Check sheet for the modelled part. Datum: model origin and axes. Units: mm. A direction names the side the tool comes from. Round coordinates to 2 decimals unless told otherwise and drop trailing zeros. Write each loop counter-clockwise with the first axis right and the second up, starting at its lowest first coordinate (ties: lowest second). Pieces come first, ordered by that corner, then holes.
Item 1: Cross-section at A-A on z = 12. Enter the section's corners in (x, y).
Item 2: Release check for a two-part mould opening along Z. For faces 1 (the flat face through (13.7, 2.8, 28.2)), 2 (the flat face through (7, 3, 0)), 3 (the flat face through (5, 0.45, 49)) record: +Z half, -Z half, draft (parallel to the pull), parting line (faces both ways), or undercut.
Item 3: Go/stop test with flat-tipped pins: pin 1 Ø0.5 at (y, z) = (0, 49) entering from +X; pin 2 Ø0.7 at (x, z) = (4.5, 43) entering from -Y; pin 3 Ø7.5 at (x, z) = (8.5, 34) entering from +Y. Record where each tip stops, or that it passes through.
Item 4: Tool access check on faces 4 (the flat face through (13.7, 2.8, 8.2)), 5 (the flat face through (6.995, -2.047, 50.675)), 6 (the flat face through (13, 2, 6.45)). Record the directions out of +Z, -Z, +X, -X, +Y, -Y that give a thin tool (end or side, any length) a straight path to the whole face; none if there is none.
Item 5: Material ranges on line 1 (Z direction, x = 12.25, y = 2.75); line 2 (Y direction, x = 11, z = 83.5); line 3 (Y direction, x = 9, z = 69), recorded low to high.
from build123d import *

# Parameters (mm, degrees)
BOSS_EXTRUDE1_DEPTH = 99.95
BOSS_EXTRUDE2_DEPTH = 99.95
SKETCH3_R           = 2.3
CUT_EXTRUDE1_DEPTH  = 203
SKETCH4_W           = 3.5
SKETCH4_H           = 4
CUT_EXTRUDE2_DEPTH  = 3
LPATTERN1_COUNT     = 10
LPATTERN1_PITCH     = 20
THICKEN1_T1         = 2
THICKEN2_T1         = 2
BOSS_EXTRUDE3_DEPTH = 99.95
CHAMFER1_SIZE       = 4.717915225
CHAMFER1_SIZE_2     = 2.2
CHAMFER2_SIZE       = 2.2


with BuildPart() as part:
    # Sketch1 → Boss-Extrude1 (new body)
    with BuildSketch(Plane.XY):
        with BuildLine():
            Line((0, 0.393921198), (0, 5.406078802))
            ThreePointArc((0, 5.406078802), (0.08229014, 5.759480212), (0.312231391, 6.040177993))
            Line((0.312231391, 6.040177993), (2.612231391, 7.809408763))
            ThreePointArc((2.612231391, 7.809408763), (3.45340141, 7.893019432), (3.9, 7.175309571))
            Line((3.9, 7.175309571), (3.9, 5.35))
            Line((3.9, 5.35), (6.3, 5.35))
            Line((6.3, 5.35), (6.3, 0.45))
            Line((6.3, 0.45), (3.9, 0.45))
            Line((3.9, 0.45), (3.9, -1.375309571))
            ThreePointArc((3.9, -1.375309571), (3.45340141, -2.093019432), (2.612231391, -2.009408763))
            Line((2.612231391, -2.009408763), (0.312231391, -0.240177993))
            ThreePointArc((0.312231391, -0.240177993), (0.08229014, 0.040519788), (0, 0.393921198))
        make_face()
    extrude(amount=BOSS_EXTRUDE1_DEPTH)

    # Sketch2 → Boss-Extrude2 (add)
    with BuildSketch(Plane.XY.offset(99.95)):
        Polygon((17.472453889, 5.35), (6.3, 5.35), (6.3, 0.45), (9.987087866, -4.283432483), (10.933774362, -3.54601491), (9.831668963, -2.122862181), (17.26318939, 3.66589025), (18.369311325, 2.245866185), (19.315997822, 2.983283759), align=None)
    extrude(amount=-BOSS_EXTRUDE2_DEPTH)

    # Sketch3 → Cut-Extrude1 (cut)
    with BuildSketch(Plane.XY.offset(99.95)):
        with Locations((9.9, 1.95)):
            Circle(SKETCH3_R)
    extrude(amount=-CUT_EXTRUDE1_DEPTH, mode=Mode.SUBTRACT)

    # Sketch4 → Cut-Extrude2 (cut)
    with BuildSketch(Plane(origin=(6.0943119, -5.034061174, 0), x_dir=(0, 0, -1), z_dir=(0.6145146443247225, -0.7889054137920846, 0))):
        with Locations((-88.2, 8.814603366)):
            Rectangle(SKETCH4_W, SKETCH4_H)
    cut_extrude2 = extrude(amount=-CUT_EXTRUDE2_DEPTH, mode=Mode.SUBTRACT)

    # LPattern1: Cut-Extrude2 ×10
    with Locations(*[(0, 0, -i * LPATTERN1_PITCH) for i in range(1, LPATTERN1_COUNT)]):
        add(cut_extrude2, mode=Mode.SUBTRACT)

    # Surface-Offset1: a surface, a copy of 1 face of the part
    surface_offset1_1 = part.part.faces().sort_by_distance((10.460431114, -3.914723696, 49.975))[0]
    add(Solid.thicken(surface_offset1_1, THICKEN1_T1))

    # Surface-Offset2: a surface, a copy of 1 face of the part
    surface_offset2_2 = part.part.faces().sort_by_distance((18.842654573, 2.614574972, 49.975))[0]
    add(Solid.thicken(surface_offset2_2, THICKEN2_T1))

    # Sketch5 → Boss-Extrude3 (add)
    with BuildSketch(Plane.XY.offset(99.95)):
        Polygon((11.216117155, -5.86124331), (9.638306327, -7.090272599), (7.794762394, -4.723556358), (9.372573222, -3.494527069), align=None)
        Polygon((22.126854473, 2.637630884), (20.28331054, 5.004347125), (17.754796681, 3.034771599), (19.598340614, 0.668055358), align=None)
    extrude(amount=-BOSS_EXTRUDE3_DEPTH)

    # Chamfer1
    # the kernel refuses this chamfer: 4.717915225, 2.2 mm, written as the material it adds along each edge
    with BuildSketch(Plane(origin=(9.372573222, -3.494527069, 99.95), x_dir=(-0.6015649261356993, 0.7988239102852083, 0), z_dir=(0, 0, -1))) as chamfer1_piece_1_section:
        Polygon((CHAMFER1_SIZE * 0.999866964139, -CHAMFER1_SIZE * 0.0163111641315), (-CHAMFER1_SIZE_2 * 0.0163111641311, -CHAMFER1_SIZE_2 * 0.999866964113), (0, 0), align=None)
    chamfer1_piece_1 = extrude(amount=99.95, mode=Mode.PRIVATE)
    chamfer1_piece_1 = split(chamfer1_piece_1, bisect_by=Plane(origin=(6.797025318, -3.442675278, 49.975), z_dir=(0.7889054137920843, 0.6145146443247225, 0)), keep=Keep.TOP, mode=Mode.PRIVATE)
    add(chamfer1_piece_1)

    # Chamfer2
    # the kernel refuses this chamfer: 2.2 mm, written as the material it adds along each edge
    with BuildSketch(Plane(origin=(18.701483177, 3.772189172, 0), x_dir=(-0.6359739526449933, 0.7717105231607922, 0), z_dir=(0, 0, 1))) as chamfer2_piece_1_section:
        Polygon((CHAMFER2_SIZE * 0.999621916911, -CHAMFER2_SIZE * 0.0274958766106), (-CHAMFER2_SIZE * 0.0274958766106, -CHAMFER2_SIZE * 0.999621916911), (0, 0), align=None)
    chamfer2_piece_1 = extrude(amount=99.95, mode=Mode.PRIVATE)
    chamfer2_piece_1 = split(chamfer2_piece_1, bisect_by=Plane(origin=(18.850985857, 5.35, 49.975), z_dir=(0, -1, 0)), keep=Keep.TOP, mode=Mode.PRIVATE)
    chamfer2_piece_1 = split(chamfer2_piece_1, bisect_by=Plane(origin=(19.861540809, 5.545809281, 49.975), z_dir=(-0.7889054137920902, -0.614514644324715, 0)), keep=Keep.TOP, mode=Mode.PRIVATE)
    add(chamfer2_piece_1)


solid = part.part
Response values:
1. outline: (0, 0.39) arc R0.8 ccw to (0.31, -0.24) - (2.61, -2.01) arc R0.8 ccw to (3.9, -1.38) - (3.9, 0.45) - (6.3, 0.45) - (6.47, 0.23) - (7.53, -4.39) - (9.64, -7.09) - (12.16, -5.12) - (10.93, -3.55) - (9.83, -2.12) - (17.26, 3.67) - (19.6, 0.67) - (22.13, 2.64) - (20.16, 5.16) - (18.62, 5.35) - (3.9, 5.35) - (3.9, 7.18) arc R0.8 ccw to (2.61, 7.81) - (0.31, 6.04) arc R0.8 ccw to (0, 5.41) - close; hole circle Ø4.6 at (9.9, 1.95)
2. face 1: undercut
2. face 2: -Z half
2. face 3: draft
3. pin 1: stops at x = 11.01
3. pin 2: stops at y = 0.45
3. pin 3: stops at y = 5.35
4. face 4: -Y
4. face 5: +Z, -Z, -Y
4. face 6: none
5. line 1: z = 0 to 6.45, 9.95 to 26.45, 29.95 to 46.45, 49.95 to 66.45, 69.95 to 86.45, 89.95 to 99.95
5. line 2: y = -6.03 to -3.63, -1.21 to -0.07, 3.97 to 5.35
5. line 3: y = -6.27 to -0.17, 4.07 to 5.35
